Geometry: final body of the model. Coordinates: model frame, mm. Face numbers are marked on the shaded views. A direction names the side the tool comes from. Round coordinates to 2 decimals unless told otherwise and drop trailing zeros. Order: outer loops, then holes, each group sorted by start corner. A loop starts at its lowest first (then second) coordinate and runs counter-clockwise, first axis right, second up. Notation, with made-up numbers: (63, -27.75) - (83, -27.75) arc R15 ccw to (83, -10.75) - close; hole circle Ø5 at (78, -31). An arc over 180 degrees is marked (long way). Put each result on its own line as item: value. Start each with the question number.
(1) Section C-C (x = 22). Output: boundary loops of the cut face in (y, z) (3 decimals).
(2) Material intervals for L1, parallel to Z at x = 29.5, y = 13; L2, parallel to X at y = 48.5, z = 45.5; L3, parallel to Z at x = -14, y = 67, sorted ascending. Write a range as [from, to].
(3) Section D-D (z = -12.5). Output: boundary loops of the cut face in (x, y), and give its area (3 significant figures).
(4) Section B-B (y = 22.5). Output: boundary loops of the cut face in (x, z), and give its area (3 significant figures).
(5) Access query for the marked faces 1 and 2. Directions: +Z, -Z, +X, -X, +Y, -Y. A direction counts if a zero-diameter tool reaches every point of the face in a straight line with its end or side. Return the directions, or none.
(6) Pin query (flat end, axial travel): P1, Ø1, axis at x = -40.5, y = 36.5, coming from the +Z side; P2, Ø5, axis at x = -19, y = 10, coming from the -Z side; P3, Ø5, axis at x = 34.5, z = 52.5, coming from the +Y side. Return the tip coordinate at first contact, or that it passes through.
(7) Section A-A (y = 68). Output: boundary loops of the cut face in (x, z).
(8) Pull-direction query (X, two-part tool) for the marked faces 3, 4, 5 and 6; classes: released by +X, released by -X, zero draft, split by the parting line, or undercut.
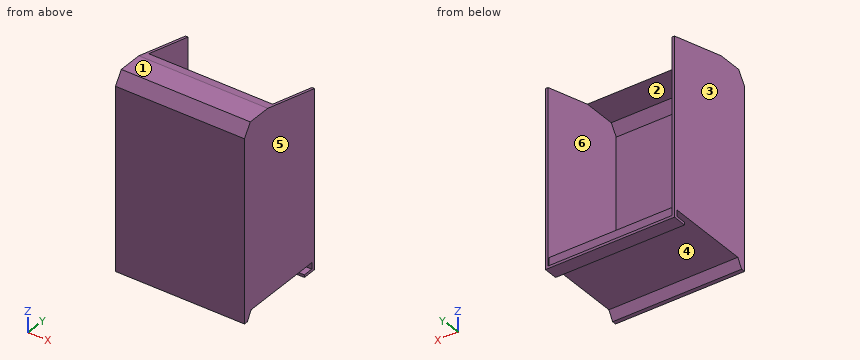
from build123d import *

# Parameters (mm, degrees)
SKETCH1_W           = 101.6
SKETCH1_H           = 152.4
BOSS_EXTRUDE1_DEPTH = 76.2
CUT_EXTRUDE1_DEPTH  = 102.6
CUT_EXTRUDE2_DEPTH  = 102.6
SHELL1_T            = -2


with BuildPart() as part:
    # Sketch1 → Boss-Extrude1 (new body)
    with BuildSketch(Plane(origin=(0, 0, 0), x_dir=(1, 0, 0), z_dir=(0, 1, 0))):
        Rectangle(SKETCH1_W, SKETCH1_H)
    extrude(amount=BOSS_EXTRUDE1_DEPTH)

    # Sketch2 → Cut-Extrude1 (cut, through all)
    with BuildSketch(Plane(origin=(50.8, 0, 0), x_dir=(0, 0, -1), z_dir=(1, 0, 0))):
        Polygon((-63.5, 76.2), (-76.2, 25.4), (-76.2, 76.2), align=None)
        Polygon((-76.2, 6.35), (-76.2, 0), (-66.675, 0), align=None)
    extrude(amount=-CUT_EXTRUDE1_DEPTH, mode=Mode.SUBTRACT)

    # Sketch3 → Cut-Extrude2 (cut, through all)
    with BuildSketch(Plane(origin=(50.8, 0, 0), x_dir=(0, 0, -1), z_dir=(1, 0, 0))):
        Polygon((69.2, 7.216451884), (69.2, 65.2), (69.2, 73.2), (74.2, 73.2), (74.2, 65.2), (76.2, 65.2), (76.2, 3.175), align=None)
    extrude(amount=-CUT_EXTRUDE2_DEPTH, mode=Mode.SUBTRACT)

    # Shell1
    shell1_openings = [part.faces().sort_by_distance(p)[0] for p in [
        (0, 76.2, -6.35),
        (0, 50.8, 69.85),
    ]]
    offset(amount=SHELL1_T, openings=shell1_openings, kind=Kind.INTERSECTION)


solid = part.part
Checks:
1. outline: (0, -76.2) - (3.175, -76.2) - (7.216, -69.2) - (73.2, -69.2) - (73.2, -74.2) - (65.2, -74.2) - (65.2, -76.2) - (76.2, -76.2) - (76.2, -74.2) - (75.2, -74.2) - (75.2, -67.2) - (6.062, -67.2) - (2.02, -74.2) - (2, -74.2) - (2, 66.069) - (7.42, 74.2) - (33.4, 74.2) - (25.4, 76.2) - (6.35, 76.2) - (0, 66.675) - close
2. L1: z = [-69.2, -67.2], [74.2, 76.2]
2. L2: x = [-50.8, -48.8], [48.8, 50.8]
2. L3: z = [-76.2, -74.2], [-69.2, -67.2]
3. outline: (-50.8, 0) - (50.8, 0) - (50.8, 76.2) - (48.8, 76.2) - (48.8, 2) - (-48.8, 2) - (-48.8, 76.2) - (-50.8, 76.2) - close
3. area: 500 mm²
4. outline: (-50.8, -69.2) - (50.8, -69.2) - (50.8, 76.2) - (-50.8, 76.2) - close; hole (-48.8, -67.2) - (48.8, -67.2) - (48.8, 74.2) - (-48.8, 74.2) - close
4. area: 972 mm²
5. face 1: +Z, +X, -X, +Y, -Y
5. face 2: +Y
6. P1: stops at z = -67.2
6. P2: stops at z = -69.2
6. P3: stops at y = 2
7. outline: (-50.8, -76.2) - (50.8, -76.2) - (50.8, -74.2) - (-50.8, -74.2) - close; (-50.8, -69.2) - (50.8, -69.2) - (50.8, 65.55) - (48.8, 65.55) - (48.8, -67.2) - (-48.8, -67.2) - (-48.8, 65.55) - (-50.8, 65.55) - close
8. face 3: released by -X
8. face 4: zero draft
8. face 5: released by +X
8. face 6: undercut
